Verification items for this drawing (mm, ordinates from the low corner). A direction names the side the tool comes from. Round coordinates to 2 decimals unless told otherwise and drop trailing zeros. Loops run counter-clockwise (first coordinate to the right, second up) from the corner with the lowest first, then second, coordinate; pieces in that order, holes last. Notation, with made-up numbers: M 9.25,-30.75 L 42.25,-30.75 A11 cw 42.25,-18.75 Z; hole C -38.75,-5 d11. An arc over 180 degrees is marked long. Answer as CSV lines item,"result".
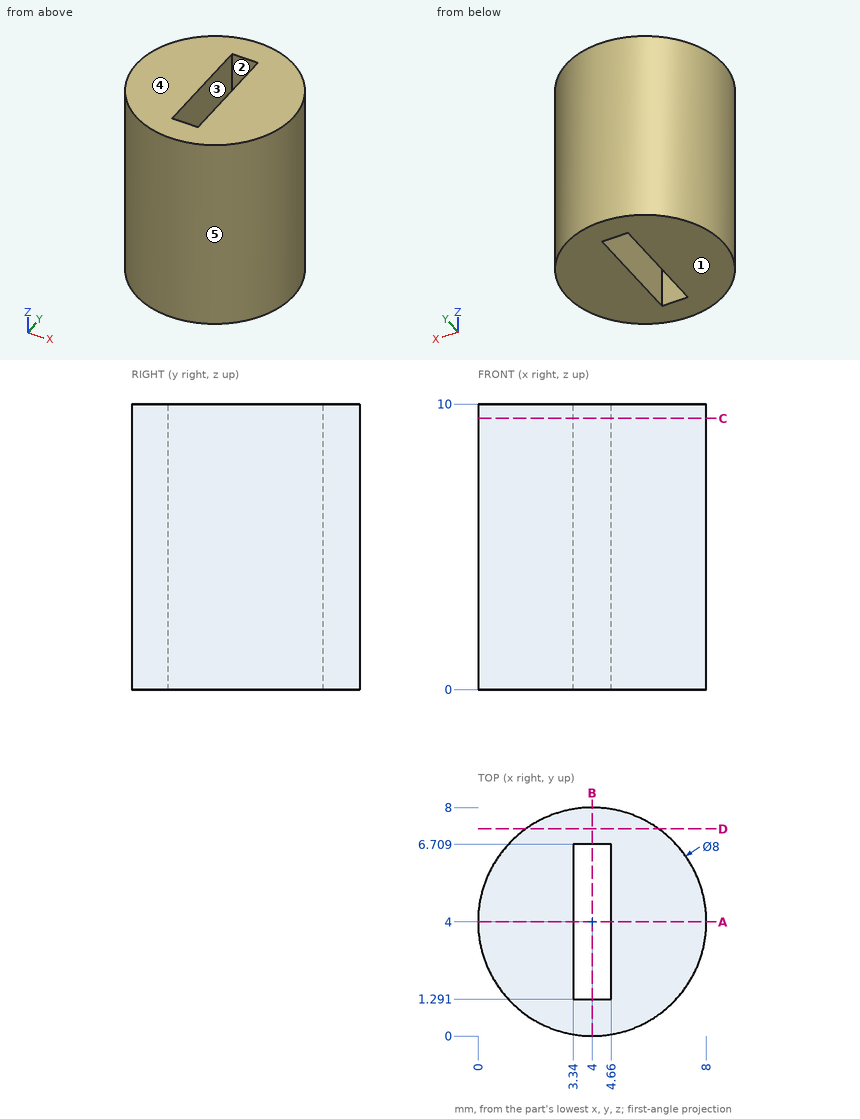
1) Draft check along X on the marked faces 3, 4 and 5. Enter one of: +X half, -X half, draft (parallel to the pull), parting line (faces both ways), or undercut.
Here are the results:
face 3,"undercut"
face 4,"draft"
face 5,"parting line"
2) Set-up check for the marked faces 1 and 2: record each of +Z, -Z, +X, -X, +Y, -Y from which the full face is reachable in a straight line by a thin tool's end or side.
Here are the results:
face 1,"-Z, +X, -X, +Y, -Y"
face 2,"+Z, -Z"
3) Section check D-D (y = 7.25). Record the cut outline in (x, z).
Here are the results:
outline,"M 1.67,0 L 6.33,0 L 6.33,10 L 1.67,10 Z"
4) Section check C-C (z = 9.5). Record the cut outline in (x, y), plus the area to 3 significant figures.
Here are the results:
outline,"C 4,4 d8; hole M 3.34,1.29 L 4.66,1.29 L 4.66,6.71 L 3.34,6.71 Z"
area,"43.1 mm^2"
5) Material ranges on probe 1 along X at (y, z) = (1.5, 6); probe 2 along X at (y, z) = (5.5, 8); probe 3 along Y at (x, z) = (3, 9.5), recorded low to high.
Here are the results:
probe 1,"x = 0.88 to 3.34, 4.66 to 7.12"
probe 2,"x = 0.29 to 3.34, 4.66 to 7.71"
probe 3,"y = 0.13 to 7.87"
6) Go/stop test with flat-tipped pins: pin 1 (1.5 mm diameter, centred on y = 2.5, z = 1.5, fed in from -X); pin 2 (3 mm diameter, centred on x = 4.5, y = 1, fed in from -Z); pin 3 (1.6 mm diameter, centred on y = 5, z = 5.5, fed in from +X) (3 decimals); pin 4 (1 mm diameter, centred on x = 5, z = 6, fed in from +Y). Record where each tip stops, or that it passes through.
Here are the results:
pin 1,"stops at x = 0.07"
pin 2,"stops at z = 0"
pin 3,"stops at x = 7.995"
pin 4,"stops at y = 7.97"
7) Section check B-B (x = 4). Record the cut outline in (y, z), plus the area to 3 significant figures.
Here are the results:
outline,"M 0,0 L 1.29,0 L 1.29,10 L 0,10 Z; M 6.71,0 L 8,0 L 8,10 L 6.71,10 Z"
area,"25.8 mm^2"
8) Section check A-A (y = 4). Record the cut outline in (x, z), plus the area to 3 significant figures.
Here are the results:
outline,"M 0,0 L 3.34,0 L 3.34,10 L 0,10 Z; M 4.66,0 L 8,0 L 8,10 L 4.66,10 Z"
area,"66.8 mm^2"
